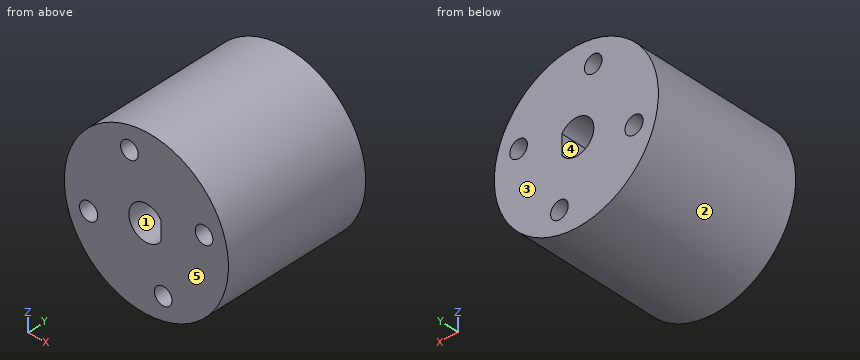
```python
from build123d import *

# Parameters (mm, degrees)
SKETCH1_R           = 13.97
SKETCH1_R_2         = 1.5
SKETCH1_R_3         = 1.543928493
BOSS_EXTRUDE1_DEPTH = 25.4
CUT_EXTRUDE1_DEPTH  = 30


with BuildPart() as part:
    # Sketch1 → Boss-Extrude1 (new body)
    with BuildSketch(Plane(origin=(0, 0, 0), x_dir=(1, 0, 0), z_dir=(0, 1, 0))):
        with Locations(Location((0, 0, 0), (0, 0, 270))):
            Circle(SKETCH1_R)
        with Locations(Location((2.876226708, 9.828189808, 0), (0, 0, 270))):
            Circle(SKETCH1_R_2, mode=Mode.SUBTRACT)
        with Locations(Location((-9.828189808, 2.876226708, 0), (0, 0, 270))):
            Circle(SKETCH1_R_3, mode=Mode.SUBTRACT)
        with Locations(Location((-2.876226708, -9.828189808, 0), (0, 0, 270))):
            Circle(SKETCH1_R_2, mode=Mode.SUBTRACT)
        with Locations(Location((9.828189808, -2.876226708, 0), (0, 0, 270))):
            Circle(SKETCH1_R_2, mode=Mode.SUBTRACT)
    extrude(amount=BOSS_EXTRUDE1_DEPTH)

    # Sketch2 → Cut-Extrude1 (cut)
    with BuildSketch(Plane(origin=(0, 25.4, 0), x_dir=(1, 0, 0), z_dir=(0, 1, 0))):
        with BuildLine():
            Line((2.465312915, -1.66), (2.465312915, 1.66))
            ThreePointArc((2.465312915, 1.66), (-2.97209821, 0), (2.465312915, -1.66))
        make_face()
    extrude(amount=-CUT_EXTRUDE1_DEPTH, mode=Mode.SUBTRACT)


solid = part.part
```
Geometry check sheet. Reference: the model listing, model coordinates, mm. Face numbers are marked on the shaded views. A direction names the side the tool comes from. Round coordinates to 2 decimals unless told otherwise and drop trailing zeros. Order: outer loops, then holes, each group sorted by start corner. A loop starts at its lowest first (then second) coordinate and runs counter-clockwise, first axis right, second up. Notation, with made-up numbers: (65, 37) - (76, 37) arc R20 cw to (76, 49) - close; hole circle Ø11 at (77.25, 26). An arc over 180 degrees is marked (long way). Use a Markdown table: item, result. Add a question column.
1) Section check B-B (x = 0). Record the cut outline in (y, z).
2) Set-up check for the marked faces 4 and 5: record each of +Z, -Z, +X, -X, +Y, -Y from which the full face is reachable in a straight line by a thin tool's end or side.
3) Section check C-C (y = 2.75). Record the cut outline in (x, z).
4) Mould release check, pull along Z, two halves, no side actions. Record for the marked faces 1, 2 and 3: released by +Z, released by -Z, zero draft, split by the parting line, or undercut.
5) Thickness scan on line 1 along X through (y, z) = (8.5, 1.5); line 2 along X through (y, z) = (22.5, 9.5); line 3 along Z through (x, y) = (-9.5, 12.75). Record the ranges inside material, lowest first.
6) Section check D-D (x = 12.25). Record the cut outline in (y, z), then the cut area to 3 significant figures.
7) Section check A-A (z = 0). Record the cut outline in (x, y).
8) Gauge pin test, flat ends, axial feed: P1, Ø1, axis at x = 3, y = 12.5, coming from the +Z side; P2, Ø3, axis at x = 10.5, y = 22.5, coming from the -Z side; P3, Ø10, axis at x = 6.5, y = 3, coming from the +Z side. Record the tip position at first contact, or that the pin passes through.
Established:
| question | item | result |
|---|---|---|
| 1 | outline | (0, -13.97) - (25.4, -13.97) - (25.4, -2.97) - (0, -2.97) - close; (0, 2.97) - (25.4, 2.97) - (25.4, 13.97) - (0, 13.97) - close |
| 2 | face 4 | +Y, -Y |
| 2 | face 5 | +Z, -Z, +X, -X, -Y |
| 3 | outline | circle Ø27.94 at (0, 0); hole circle Ø3.09 at (-9.83, -2.88); hole circle Ø3 at (-2.88, 9.83); hole circle Ø3 at (2.88, -9.83); hole (2.47, -1.66) - (2.47, 1.66) arc R2.97 ccw (long way) to start; hole circle Ø3 at (9.83, 2.88) |
| 4 | face 1 | undercut |
| 4 | face 2 | split by the parting line |
| 4 | face 3 | zero draft |
| 5 | line 1 | -13.89 to -2.57, 2.47 to 9.23, 10.42 to 13.89 |
| 5 | line 2 | -10.24 to -4.34, -1.41 to 10.24 |
| 5 | line 3 | -10.24 to -4.38, -1.37 to 10.24 |
| 6 | outline | (0, -6.72) - (25.4, -6.72) - (25.4, 6.72) - (0, 6.72) - close |
| 6 | area | 341 mm2 |
| 7 | outline | (-13.97, 0) - (-2.97, 0) - (-2.97, 25.4) - (-13.97, 25.4) - close; (2.47, 0) - (13.97, 0) - (13.97, 25.4) - (2.47, 25.4) - close |
| 8 | P1 | z = 13.74 |
| 8 | P2 | z = -10.68 |
| 8 | P3 | z = 13.89 |
